Can you work these out from the drawing? Everything is in mm from the part's minimum corner. A direction names the side the tool comes from. Coordinates: 2 decimals unless noted, no trailing zeros. Loops run counter-clockwise (first coordinate to the right, second up) from the corner with the lowest first, then second, coordinate; pieces in that order, holes last. Notation, with made-up numbers: M 83.25,54 L 117.25,54 A30 ccw 117.25,93 Z; hole C -22.75,-37.75 d5. An arc over 180 degrees is marked long. Use CSV: the item, a comma, the result in double quotes. Start each with the question number.
Q1. If we section it at B-B (x = 68.55): Please give me the cut outline in (y, z).
Q2. Which directions (+Z, -Z, +X, -X, +Y, -Y) give clear straight access to the entire face, cutting with the end or side of a thin tool? Please do the marked faces 1, 2 and 3.
Q3. For pin 1 Ø4 at (x, y) = (68.55, 21.45) entering from +Z; pin 2 Ø6.5 at (x, y) = (21.45, 21.45) entering from +Z; pin 3 Ø3 at (x, z) = (79, 43.5) entering from -Y; pin 4 Ø6.5 at (x, z) = (84, 59.5) entering from -Y, each with a flat end and sliding along its axis, tell me the tip position at first contact or that it passes through.
Q4. If we section it at D-D (y = 68.55): Please give me the cut outline in (x, z), and give its area (3 significant figures).
Q5. If we mould it in two halves opening along X, with no side actions, what happens to the marked faces 4, 5 and 6? For each: +X half, -X half, draft (parallel to the pull), parting line (faces both ways), or undercut.
Q6. If we section it at C-C (z = 14): Please give me the cut outline in (x, y).
Q7. Please list where these lines run through material, in increasing order: probe 1 along Y at (x, z) = (45, 2.25); probe 2 along X at (y, z) = (8, 12.5); probe 3 along Y at (x, z) = (68.55, 2.75). Write a range as [from, to].
Q8. If we section it at A-A (x = 6): Please give me the cut outline in (y, z) (1 decimal).
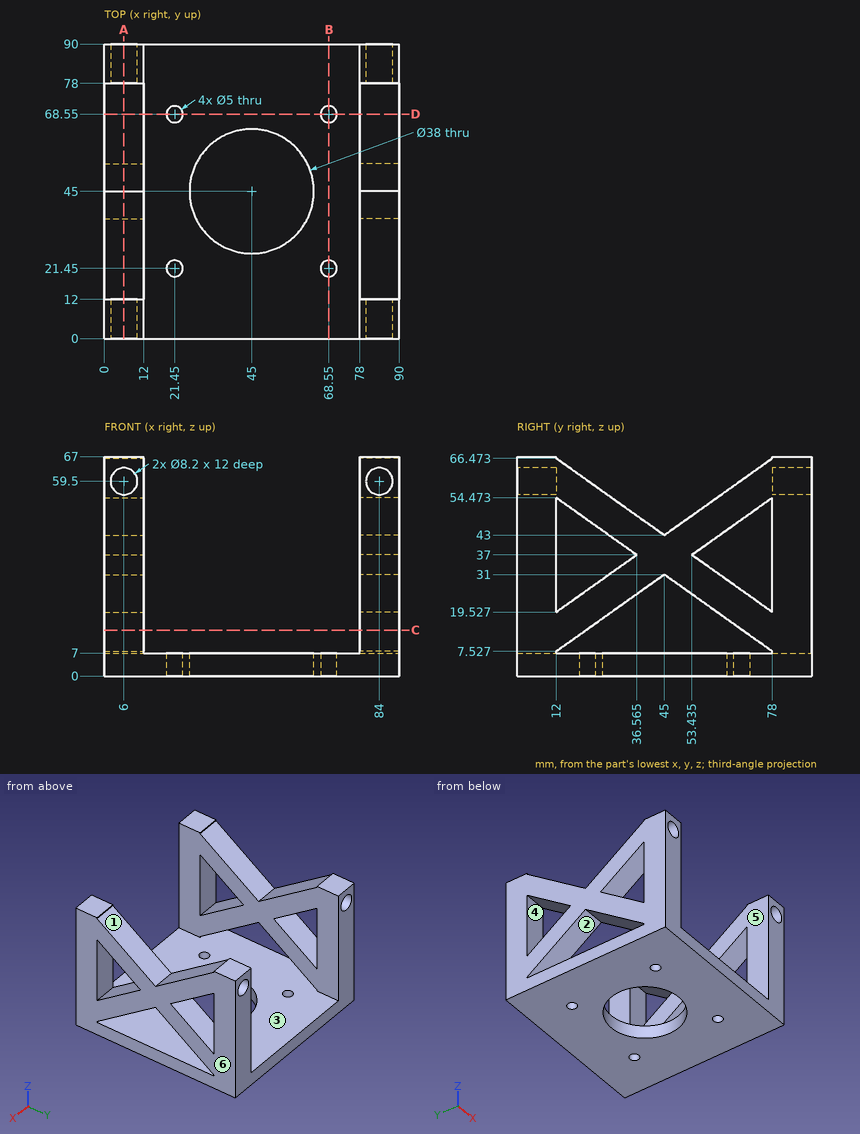
Results below:
1,outline,"M 0,0 L 18.95,0 L 18.95,7 L 0,7 Z; M 23.95,0 L 66.05,0 L 66.05,7 L 23.95,7 Z; M 71.05,0 L 90,0 L 90,7 L 71.05,7 Z"
2,face 1,"+Z, +X, -X"
2,face 2,"+X, -X"
2,face 3,"none"
3,pin 1,"through"
3,pin 2,"z = 7"
3,pin 3,"y = 0"
3,pin 4,"y = 12"
4,outline,"M 0,0 L 18.95,0 L 18.95,7 L 0,7 Z; M 0,14.25 L 12,14.25 L 12,26.25 L 0,26.25 Z; M 0,47.75 L 12,47.75 L 12,59.75 L 0,59.75 Z; M 23.95,0 L 66.05,0 L 66.05,7 L 23.95,7 Z; M 71.05,0 L 90,0 L 90,7 L 71.05,7 Z; M 78,14.25 L 90,14.25 L 90,26.25 L 78,26.25 Z; M 78,47.75 L 90,47.75 L 90,59.75 L 78,59.75 Z"
4,area,"1,140 mm^2"
5,face 4,"draft"
5,face 5,"undercut"
5,face 6,"+X half"
6,outline,"M 0,0 L 12,0 L 12,21.1 L 0,21.1 Z; M 0,68.9 L 12,68.9 L 12,90 L 0,90 Z; M 78,0 L 90,0 L 90,21.1 L 78,21.1 Z; M 78,68.9 L 90,68.9 L 90,90 L 78,90 Z"
7,probe 1,"[0, 26], [64, 90]"
7,probe 2,"[0, 12], [78, 90]"
7,probe 3,"[0, 18.95], [23.95, 66.05], [71.05, 90]"
8,outline,"M 0,0 L 90,0 L 90,55.4 L 78,55.4 L 78,63.6 L 90,63.6 L 90,67 L 78,67 L 78,66.5 L 45,43 L 12,66.5 L 12,67 L 0,67 L 0,63.6 L 12,63.6 L 12,55.4 L 0,55.4 Z; hole M 12,7 L 78,7 L 78,7.5 L 45,31 L 12,7.5 Z; hole M 12,19.5 L 36.6,37 L 12,54.5 Z; hole M 53.4,37 L 78,19.5 L 78,54.5 Z"
